Read the model definition and answer for the solid it produces. Units are mm, in the model's axes. A direction names the side the tool comes from. Coordinates: 2 decimals unless noted, no trailing zeros.
1) Which of the six approach directions +Z, -Z, +X, -X, +Y, -Y give full straight-line access (tool end or side, diameter ignored) to faces 1 (the face through (-36.18, 7.553, 0.11)), 2 (the face through (-39.729, -7, 0))?
2) Find the intervals of material crossed by line 1 (Y direction, x = 23, z = -2); line 2 (X direction, y = 17, z = -0.75); line 3 (Y direction, x = -17.5, z = 2.25), in increasing order.
3) Each of these flat-tipped pins is pushed along its axis until it touches: pin 1 Ø1 at (y, z) = (5, 2) entering from +X; pin 2 Ø4 at (y, z) = (0.5, -3.5) entering from +X; pin 3 Ø4 at (x, z) = (17.5, 3) entering from -Y. Where does it stop, or does it pass through?
4) Determine the mould class of faces 3 (the face through (-36.18, -4.947, 0.11)), 4 (the face through (-39.729, 5, 0)) for opening direction Y: +Y half, -Y half, draft (parallel to the pull), parting line (faces both ways), or undercut.
from build123d import *

# Parameters (mm, degrees)
EXTRUDE_1_DEPTH      = 5
EXTRUDE_1_DEPTH_BACK = 5
FILLET_3_R           = 5
SKETCH_2_R           = 2.5
EXTRUDE_2_DEPTH      = 7


with BuildPart() as part:
    # 草圖1 → 填料-伸長1 (new, two sides: drawn at the far end of the back side and taken through both)
    with BuildSketch(Plane.XY.offset(-EXTRUDE_1_DEPTH_BACK)):
        with BuildLine():
            Line((-32.728711913, 18.847882673), (-32.728711913, -16.152117327))
            add(Edge.make_bspline(
                [(-32.728711913, -16.152117327), (-21.783034561, -22.826167416), (-15.535655433, -11.364162116)],
                knots=[0, 0, 0, 1, 1, 1], degree=2))
            add(Edge.make_bspline(
                [(-15.535655433, -11.364162116), (-4.773052761, -12.557057066), (-4.030638728, -2.071536696)],
                knots=[0, 0, 0, 1, 1, 1], degree=2))
            add(Edge.make_bspline(
                [(5.051083958, 8.507759935), (4.922923736, -0.27289527), (-4.030638728, -2.071536696)],
                knots=[0, 0, 0, 1, 1, 1], degree=2))
            add(Edge.make_bspline(
                [(17.917796077, 23.375960607), (18.197143612, 10.254572471), (5.051083958, 8.507759935)],
                knots=[0, 0, 0, 1, 1, 1], degree=2))
            add(Edge.make_bspline(
                [(31.447225321, 54.936813216), (37.191964726, 29.582174335), (17.917796077, 23.375960607)],
                knots=[0, 0, 0, 1, 1, 1], degree=2))
            add(Edge.make_bspline(
                [(-32.728711913, 18.847882673), (5.094383594, 25.874030711), (31.447225321, 54.936813216)],
                knots=[0, 0, 0, 1, 1, 1], degree=2))
        make_face()
    extrude(amount=EXTRUDE_1_DEPTH + EXTRUDE_1_DEPTH_BACK)

    # 圓角3
    fillet_3_edges = [part.edges().sort_by_distance(p)[0] for p in [
        (2.226820149, 31.383189328, -5),
        (2.226820149, 31.383189328, 5),
    ]]
    fillet(fillet_3_edges, radius=FILLET_3_R - 0.0001)  # a hair under: the kernel refuses the full size

    # 草圖2 → 填料-伸長2 (add)
    with BuildSketch(Plane.ZY.offset(32.728711913)):
        with Locations(Location((0, 5.055113449, 0), (0, 0, 270))):
            Circle(SKETCH_2_R)
        with Locations(Location((0, -7.444886551, 0), (0, 0, 270))):
            Circle(SKETCH_2_R)
    extrude(amount=EXTRUDE_2_DEPTH)


solid = part.part
Reported:
1. face 1: -X
1. face 2: +Z, -Z, -X, +Y, -Y
2. line 1: y = 25.59 to 45.89
2. line 2: x = -32.73 to 17.05
2. line 3: y = -14.38 to 22.16
3. pin 1: stops at x = 4.7
3. pin 2: stops at x = 3.47
3. pin 3: stops at y = 13.94
4. face 3: undercut
4. face 4: draft
